Verification items for the finished model (mm, model axes). Face numbers are marked on the shaded views. Round coordinates to 2 decimals unless told otherwise and drop trailing zeros. Order: outer loops, then holes, each group sorted by start corner. A loop starts at its lowest first (then second) coordinate and runs counter-clockwise, first axis right, second up. Notation, with made-up numbers: M -4,16 L 37,16 A5 cw 37,23 Z; hole C 80.25,15.25 d1. An arc over 180 degrees is marked long. One line per item, written item: value. Start each with the question number.
from build123d import *

# Parameters (mm, degrees)
SKETCH3_W           = 65
SKETCH3_H           = 60
BOSS_EXTRUDE3_DEPTH = 5
SKETCH5_W           = 43
SKETCH5_H           = 35
CUT_EXTRUDE2_DEPTH  = 10
CUT_EXTRUDE1_REACH  = 57.982
SKETCH4_R           = 1.3
SKETCH9_R           = 2.65
SKETCH9_R_2         = 1.05
BOSS_EXTRUDE5_DEPTH = 6


with BuildPart() as part:
    # Sketch3 → Boss-Extrude3 (new body)
    with BuildSketch(Plane(origin=(0, 0, 0), x_dir=(1, 0, 0), z_dir=(0, 1, 0))):
        with Locations((-14.5, 0)):
            Rectangle(SKETCH3_W, SKETCH3_H)
    extrude(amount=BOSS_EXTRUDE3_DEPTH)

    # Sketch5 → Cut-Extrude2 (cut)
    with BuildSketch(Plane.XZ):
        with Locations((-14.5, 0)):
            Rectangle(SKETCH5_W, SKETCH5_H)
    extrude(amount=-CUT_EXTRUDE2_DEPTH, mode=Mode.SUBTRACT)

    # Sketch4 → Cut-Extrude1 (cut, up to next)
    with BuildSketch(Plane(origin=(0, 5, 0), x_dir=(1, 0, 0), z_dir=(0, 1, 0)), mode=Mode.PRIVATE) as cut_extrude1_sk1:
        with Locations(Location((-33.5, 20, 0), (0, 0, 270))):
            Circle(SKETCH4_R)
    cut_extrude1_tool1 = extrude(cut_extrude1_sk1.sketch, amount=-CUT_EXTRUDE1_REACH, mode=Mode.PRIVATE) & part.part
    # Sketch4 → Cut-Extrude1 (cut, up to next)
    with BuildSketch(Plane(origin=(0, 5, 0), x_dir=(1, 0, 0), z_dir=(0, 1, 0)), mode=Mode.PRIVATE) as cut_extrude1_sk2:
        with Locations(Location((4.5, 20, 0), (0, 0, 270))):
            Circle(SKETCH4_R)
    cut_extrude1_tool2 = extrude(cut_extrude1_sk2.sketch, amount=-CUT_EXTRUDE1_REACH, mode=Mode.PRIVATE) & part.part
    # Sketch4 → Cut-Extrude1 (cut, up to next)
    with BuildSketch(Plane(origin=(0, 5, 0), x_dir=(1, 0, 0), z_dir=(0, 1, 0)), mode=Mode.PRIVATE) as cut_extrude1_sk3:
        with Locations(Location((4.5, -20, 0), (0, 0, 270))):
            Circle(SKETCH4_R)
    cut_extrude1_tool3 = extrude(cut_extrude1_sk3.sketch, amount=-CUT_EXTRUDE1_REACH, mode=Mode.PRIVATE) & part.part
    # Sketch4 → Cut-Extrude1 (cut, up to next)
    with BuildSketch(Plane(origin=(0, 5, 0), x_dir=(1, 0, 0), z_dir=(0, 1, 0)), mode=Mode.PRIVATE) as cut_extrude1_sk4:
        with Locations(Location((-33.5, -20, 0), (0, 0, 270))):
            Circle(SKETCH4_R)
    cut_extrude1_tool4 = extrude(cut_extrude1_sk4.sketch, amount=-CUT_EXTRUDE1_REACH, mode=Mode.PRIVATE) & part.part
    add(cut_extrude1_tool1.solids().sort_by_distance((-33.5, 5, -20))[0], mode=Mode.SUBTRACT)
    add(cut_extrude1_tool2.solids().sort_by_distance((4.5, 5, -20))[0], mode=Mode.SUBTRACT)
    add(cut_extrude1_tool3.solids().sort_by_distance((4.5, 5, 20))[0], mode=Mode.SUBTRACT)
    add(cut_extrude1_tool4.solids().sort_by_distance((-33.5, 5, 20))[0], mode=Mode.SUBTRACT)

    # Sketch9 → Boss-Extrude5 (add)
    # profile 1 of 4: a face of its own
    with BuildSketch(Plane.XZ):
        with Locations(Location((-33.5, 20, 0), (0, 0, 250.629961754))):
            Circle(SKETCH9_R)
        with Locations(Location((-33.5, 20, 0), (0, 0, 270))):
            Circle(SKETCH9_R_2, mode=Mode.SUBTRACT)
    # profile 2 of 4: a face of its own
    with BuildSketch(Plane.XZ):
        with Locations(Location((-33.5, -20, 0), (0, 0, 109.370038246))):
            Circle(SKETCH9_R)
        with Locations(Location((-33.5, -20, 0), (0, 0, 270))):
            Circle(SKETCH9_R_2, mode=Mode.SUBTRACT)
    # profile 3 of 4: a face of its own
    with BuildSketch(Plane.XZ):
        with Locations(Location((4.5, 20, 0), (0, 0, 289.370038246))):
            Circle(SKETCH9_R)
        with Locations(Location((4.5, 20, 0), (0, 0, 270))):
            Circle(SKETCH9_R_2, mode=Mode.SUBTRACT)
    # profile 4 of 4: a face of its own
    with BuildSketch(Plane.XZ):
        with Locations(Location((4.5, -20, 0), (0, 0, 109.370038246))):
            Circle(SKETCH9_R)
        with Locations(Location((4.5, -20, 0), (0, 0, 270))):
            Circle(SKETCH9_R_2, mode=Mode.SUBTRACT)
    extrude(amount=BOSS_EXTRUDE5_DEPTH)


solid = part.part
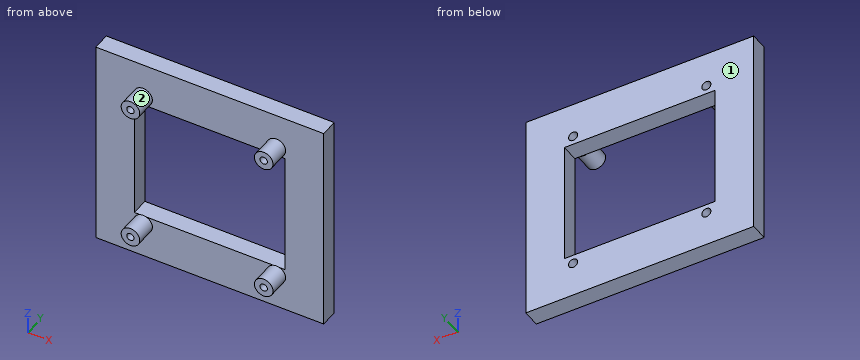
1. Section check B-B (z = 20). Record the cut outline in (x, y).
2. Section check D-D (x = -33.5). Give the number of separate pieces and of enclosed holes in the cut face, and give its area (3 significant figures).
3. Scan lines: line 1 along X through (y, z) = (-4.65, -20); line 2 along X through (y, z) = (4.25, 3); line 3 along X through (y, z) = (2.9, -20). Record each from-to range of solid material in increasing order.
4. Draft check along X on the marked faces 1 and 2. Enter one of: released by +X, released by -X, zero draft, split by the parting line, or undercut.
5. Section check C-C (x = -20.5). Record the cut outline in (y, z), and give its area (3 significant figures).
6. Section check A-A (y = -4.25). Record the cut outline in (x, z), and give its area (3 significant figures).
7. Depth check by flat-ended pin: pin 1 (2.5 mm diameter, centred on x = -33.5, z = -20, fed in from +Y). Enter the tip coordinate at first touch or a pass-through.
Geometry check:
1. outline: M -47,0 L -36.15,0 L -36.15,-6 L -34.55,-6 L -34.55,0 L -34.8,0 L -34.8,5 L -47,5 Z; M -32.45,-6 L -30.85,-6 L -30.85,0 L 1.85,0 L 1.85,-6 L 3.45,-6 L 3.45,0 L 3.2,0 L 3.2,5 L -32.2,5 L -32.2,0 L -32.45,0 Z; M 5.55,-6 L 7.15,-6 L 7.15,0 L 18,0 L 18,5 L 5.8,5 L 5.8,0 L 5.55,0 Z
2. separate pieces: 4
2. enclosed holes: 0
2. area: 137 mm²
3. line 1: x = -36.15 to -34.55, -32.45 to -30.85, 1.85 to 3.45, 5.55 to 7.15
3. line 2: x = -47 to -36, 7 to 18
3. line 3: x = -47 to -34.8, -32.2 to 3.2, 5.8 to 18
4. face 1: zero draft
4. face 2: undercut
5. outline: M 0,-30 L 5,-30 L 5,-17.5 L 0,-17.5 Z; M 0,17.5 L 5,17.5 L 5,30 L 0,30 Z
5. area: 125 mm²
6. outline: C -33.5,-20 d5.3; C -33.5,20 d5.3; C 4.5,-20 d5.3; C 4.5,20 d5.3; hole C -33.5,-20 d2.1; hole C -33.5,20 d2.1; hole C 4.5,-20 d2.1; hole C 4.5,20 d2.1
6. area: 74.4 mm²
7. pin 1: stops at y = 0
